The listing builds one solid part. Answer for the finished solid, in the listing's coordinates (mm). Coordinates: 2 decimals unless noted, no trailing zeros. Order: outer loops, then holes, each group sorted by start corner. A loop starts at its lowest first (then second) coordinate and runs counter-clockwise, first axis right, second up. Notation, with made-up numbers: (-5.75, 67.25) -> (29.25, 67.25) arc R21 cw to (29.25, 81.25) -> close; hole circle Ø8 at (23, 27.25). An arc over 180 degrees is marked (long way). Put each result on its own line as item: value. Start each with the question number.
```python
from build123d import *

# Parameters (mm, degrees)
SKETCH1_W           = 245
SKETCH1_H           = 200
BOSS_EXTRUDE1_DEPTH = 6
SKETCH2_W           = 245
SKETCH2_H           = 200
SKETCH2_W_2         = 220.5
SKETCH2_H_2         = 180
BOSS_EXTRUDE2_DEPTH = 80
SKETCH3_W           = 3
SKETCH3_H           = 180
BOSS_EXTRUDE3_DEPTH = 75
SKETCH5_W           = 230.5
SKETCH5_H           = 190
SKETCH5_W_2         = 220.5
SKETCH5_H_2         = 180
CUT_EXTRUDE1_DEPTH  = 5
SKETCH6_R           = 11.65
CUT_EXTRUDE2_DEPTH  = 3
FILLET1_R           = 5
FILLET2_R           = 2


with BuildPart() as part:
    # Sketch1 → Boss-Extrude1 (new body)
    with BuildSketch(Plane.XY):
        Rectangle(SKETCH1_W, SKETCH1_H)
    extrude(amount=BOSS_EXTRUDE1_DEPTH)

    # Sketch2 → Boss-Extrude2 (add)
    with BuildSketch(Plane.XY.offset(6)):
        Rectangle(SKETCH2_W, SKETCH2_H)
        Rectangle(SKETCH2_W_2, SKETCH2_H_2, mode=Mode.SUBTRACT)
    extrude(amount=BOSS_EXTRUDE2_DEPTH)

    # Sketch3 → Boss-Extrude3 (add)
    with BuildSketch(Plane.XY.offset(6)):
        Rectangle(SKETCH3_W, SKETCH3_H)
    extrude(amount=BOSS_EXTRUDE3_DEPTH)

    # Sketch5 → Cut-Extrude1 (cut)
    with BuildSketch(Plane.XY.offset(86)):
        Rectangle(SKETCH5_W, SKETCH5_H)
        Rectangle(SKETCH5_W_2, SKETCH5_H_2, mode=Mode.SUBTRACT)
    extrude(amount=-CUT_EXTRUDE1_DEPTH, mode=Mode.SUBTRACT)

    # Sketch6 → Cut-Extrude2 (cut)
    with BuildSketch(Plane.XY.offset(6)):
        with Locations((16.29, 54)):
            Circle(SKETCH6_R)
        with Locations((42.68, 54)):
            Circle(SKETCH6_R)
        with Locations((69.07, 54)):
            Circle(SKETCH6_R)
        with Locations((95.46, 54)):
            Circle(SKETCH6_R)
        with Locations((16.29, 18)):
            Circle(SKETCH6_R)
        with Locations((42.68, 18)):
            Circle(SKETCH6_R)
        with Locations((69.07, 18)):
            Circle(SKETCH6_R)
        with Locations((95.46, 18)):
            Circle(SKETCH6_R)
        with Locations((16.29, -18)):
            Circle(SKETCH6_R)
        with Locations((42.68, -18)):
            Circle(SKETCH6_R)
        with Locations((69.07, -18)):
            Circle(SKETCH6_R)
        with Locations((95.46, -18)):
            Circle(SKETCH6_R)
        with Locations((16.29, -54)):
            Circle(SKETCH6_R)
        with Locations((42.68, -54)):
            Circle(SKETCH6_R)
        with Locations((69.07, -54)):
            Circle(SKETCH6_R)
        with Locations((95.46, -54)):
            Circle(SKETCH6_R)
        with Locations(Location((-95.46, -54, 0), (0, 0, 180))):
            Circle(SKETCH6_R)
        with Locations(Location((-69.07, -54, 0), (0, 0, 180))):
            Circle(SKETCH6_R)
        with Locations(Location((-42.68, -54, 0), (0, 0, 180))):
            Circle(SKETCH6_R)
        with Locations(Location((-16.29, -54, 0), (0, 0, 180))):
            Circle(SKETCH6_R)
        with Locations(Location((-95.46, -18, 0), (0, 0, 180))):
            Circle(SKETCH6_R)
        with Locations(Location((-69.07, -18, 0), (0, 0, 180))):
            Circle(SKETCH6_R)
        with Locations(Location((-42.68, -18, 0), (0, 0, 180))):
            Circle(SKETCH6_R)
        with Locations(Location((-16.29, -18, 0), (0, 0, 180))):
            Circle(SKETCH6_R)
        with Locations(Location((-95.46, 18, 0), (0, 0, 180))):
            Circle(SKETCH6_R)
        with Locations(Location((-69.07, 18, 0), (0, 0, 180))):
            Circle(SKETCH6_R)
        with Locations(Location((-42.68, 18, 0), (0, 0, 180))):
            Circle(SKETCH6_R)
        with Locations(Location((-16.29, 18, 0), (0, 0, 180))):
            Circle(SKETCH6_R)
        with Locations(Location((-95.46, 54, 0), (0, 0, 180))):
            Circle(SKETCH6_R)
        with Locations(Location((-69.07, 54, 0), (0, 0, 180))):
            Circle(SKETCH6_R)
        with Locations(Location((-42.68, 54, 0), (0, 0, 180))):
            Circle(SKETCH6_R)
        with Locations(Location((-16.29, 54, 0), (0, 0, 180))):
            Circle(SKETCH6_R)
    extrude(amount=-CUT_EXTRUDE2_DEPTH, mode=Mode.SUBTRACT)

    # Fillet1
    fillet1_edges = [part.edges().sort_by_distance(p)[0] for p in [
        (122.5, 0, 86),
        (0, 100, 86),
        (-122.5, 0, 86),
        (0, -100, 86),
        (0, 100, 0),
        (122.5, 0, 0),
        (0, -100, 0),
        (-122.5, 0, 0),
        (-122.5, 100, 43),
        (122.5, 100, 43),
        (122.5, -100, 43),
        (-122.5, -100, 43),
    ]]
    fillet(fillet1_edges, radius=FILLET1_R - 0.0001)  # a hair under: the kernel refuses the full size

    # Fillet2
    fillet2_edges = [part.edges().sort_by_distance(p)[0] for p in [
        (1.5, -90, 43.5),
        (1.5, 90, 43.5),
        (-1.5, 90, 43.5),
        (-1.5, -90, 43.5),
        (-110.25, 90, 43.5),
        (-110.25, -90, 43.5),
        (110.25, -90, 43.5),
        (110.25, 90, 43.5),
    ]]
    fillet(fillet2_edges, radius=FILLET2_R)


solid = part.part
```
(1) Find the intervals of material crossed by L1, parallel to X at y = 36.5, z = 78.5; L2, parallel to Y at x = -69.07, z = 5; L3, parallel to Y at x = 61, z = 24, in increasing order.
(2) For a pull along Y with two mould halves and no side action, classify faces 1 (the cylindrical face through (-121.07, 1.33, 84.5)), 2 (the cylindrical face through (-121.07, -98.5, 43.53)), 3 (the flat face through (16, 18, 3)) as released by +Y, released by -Y, zero draft, split by the parting line, or undercut.
(3) The part is cut by section A-A on z = 20.5. Determine the outline of the cut face in (x, y).
(4) The part is cut by section C-C on y = 37. Determine the outline of the cut face in (x, z), plus the area to 3 significant figures.
(5) Each of these flat-tipped pins is pushed along its axis until it touches: P1, Ø7, axis at x = 100, y = 20.5, coming from the +Z side; P2, Ø18.5, axis at x = 99, y = -23.5, coming from the +Z side. Where does it stop, or does it pass through?
Worked out:
1. L1: -122.5 to -110.25, -1.5 to 1.5, 110.25 to 122.5
1. L2: -100 to -65.65, -42.35 to -29.65, -6.35 to 6.35, 29.65 to 42.35, 65.65 to 100
1. L3: -100 to -90, 90 to 100
2. face 1: zero draft
2. face 2: released by -Y
2. face 3: undercut
3. outline: (-122.5, -95) arc R5 ccw to (-117.5, -100) -> (117.5, -100) arc R5 ccw to (122.5, -95) -> (122.5, 95) arc R5 ccw to (117.5, 100) -> (-117.5, 100) arc R5 ccw to (-122.5, 95) -> close; hole (-110.25, -88) arc R2 ccw to (-108.25, -90) -> (-3.5, -90) arc R2 ccw to (-1.5, -88) -> (-1.5, 88) arc R2 ccw to (-3.5, 90) -> (-108.25, 90) arc R2 ccw to (-110.25, 88) -> close; hole (1.5, -88) arc R2 ccw to (3.5, -90) -> (108.25, -90) arc R2 ccw to (110.25, -88) -> (110.25, 88) arc R2 ccw to (108.25, 90) -> (3.5, 90) arc R2 ccw to (1.5, 88) -> close
4. outline: (-122.5, 5) arc R5 ccw to (-117.5, 0) -> (117.5, 0) arc R5 ccw to (122.5, 5) -> (122.5, 81) arc R5 ccw to (117.5, 86) -> (115.25, 86) -> (115.25, 81) -> (110.25, 81) -> (110.25, 6) -> (1.5, 6) -> (1.5, 81) -> (-1.5, 81) -> (-1.5, 6) -> (-110.25, 6) -> (-110.25, 81) -> (-115.25, 81) -> (-115.25, 86) -> (-117.5, 86) arc R5 ccw to (-122.5, 81) -> close
4. area: 3,580 mm2
5. P1: z = 3
5. P2: z = 6
